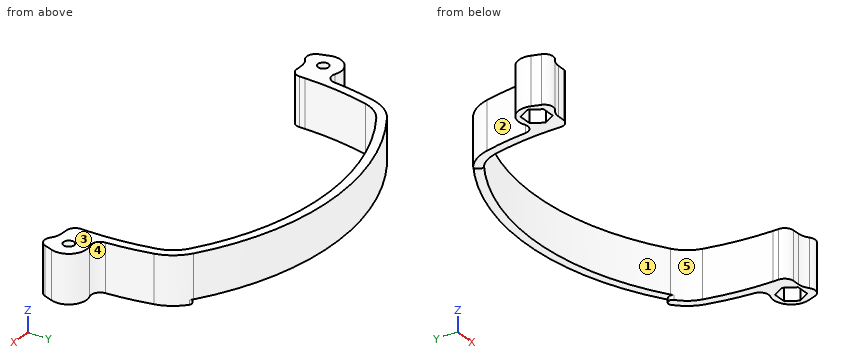
from build123d import *

# Parameters (mm, degrees)
BOSS_EXTRUDE1_DEPTH   = 17.145
BOSS_EXTRUDE2_START   = -17.145
BOSS_EXTRUDE2_DEPTH   = 17.145
F_6_CLEARANCE_HOLE3_D = 3.7973
CUT_EXTRUDE2_DEPTH    = 6.35
FILLET1_R             = 3.175
CUT_EXTRUDE3_DEPTH    = 1.5875
FILLET2_R             = 1.27


with BuildPart() as part:
    # Sketch1 → Boss-Extrude1 (new body)
    with BuildSketch(Plane.XY):
        with BuildLine():
            Line((-60.325, -44.9072), (-57.15, -44.9072))
            ThreePointArc((-57.15, -44.9072), (-56.454091105, -33.036041743), (-54.37589767, -21.327506412))
            ThreePointArc((-54.37589767, -21.327506412), (-52.38952724, -16.938887877), (-48.911621193, -13.605749768))
            ThreePointArc((-48.911621193, -13.605749768), (0, 0.8128), (48.911621193, -13.605749768))
            ThreePointArc((48.911621193, -13.605749768), (52.38952724, -16.938887877), (54.37589767, -21.327506412))
            ThreePointArc((54.37589767, -21.327506412), (56.454091105, -33.036041743), (57.15, -44.9072))
            Line((57.15, -44.9072), (60.325, -44.9072))
            ThreePointArc((60.325, -44.9072), (59.607343952, -32.665068047), (57.464206972, -20.590640987))
            ThreePointArc((57.464206972, -20.590640987), (54.981243935, -15.104867818), (50.633861375, -10.938445182))
            ThreePointArc((50.633861375, -10.938445182), (0, 3.9878), (-50.633861375, -10.938445182))
            ThreePointArc((-50.633861375, -10.938445182), (-54.981243935, -15.104867818), (-57.464206972, -20.590640987))
            ThreePointArc((-57.464206972, -20.590640987), (-59.607343952, -32.665068047), (-60.325, -44.9072))
        make_face()
    extrude(amount=BOSS_EXTRUDE1_DEPTH)

    # Sketch5 → Boss-Extrude2 (add)
    with BuildSketch(Plane.XY.offset(17.145).offset(BOSS_EXTRUDE2_START)):
        with BuildLine():
            Line((-72.692160527, -46.93606155), (-71.648700283, -50.030736885))
            ThreePointArc((-71.648700283, -50.030736885), (-69.548845385, -52.05848349), (-66.680845425, -51.514679193))
            ThreePointArc((-66.680845425, -51.514679193), (-64.835115794, -50.509265825), (-62.762296236, -50.16142536))
            Line((-62.762296236, -50.16142536), (-60.304367197, -50.16142536))
            ThreePointArc((-60.304367197, -50.16142536), (-58.037136322, -49.209101486), (-57.129992434, -46.923418531))
            ThreePointArc((-57.129992434, -46.923418531), (-57.144997985, -45.9153589), (-57.15, -44.9072))
            Line((-57.15, -44.9072), (-60.325, -44.9072))
            ThreePointArc((-60.325, -44.9072), (-67.702990917, -38.640962319), (-72.692160527, -46.93606155))
        make_face()
    boss_extrude2 = extrude(amount=BOSS_EXTRUDE2_DEPTH)

    # #6 Clearance Hole3 (through all)
    with Locations(Plane(origin=(0, 0, 0), x_dir=(-1, 0, 0), z_dir=(0, 0, -1))):
        with Locations((66.675, -44.9072)):
            f_6_clearance_hole3 = Hole(F_6_CLEARANCE_HOLE3_D / 2)

    # Sketch9 → Cut-Extrude2 (cut)
    with BuildSketch(Plane(origin=(0, 0, 0), x_dir=(-1, 0, 0), z_dir=(0, 0, -1))):
        Polygon((69.076344107, -40.74795), (64.273655893, -40.74795), (61.872311786, -44.9072), (64.273655893, -49.06645), (69.076344107, -49.06645), (71.477688214, -44.9072), align=None)
    cut_extrude2 = extrude(amount=-CUT_EXTRUDE2_DEPTH, mode=Mode.SUBTRACT)

    # Mirror1: Boss-Extrude2, #6 Clearance Hole3, Cut-Extrude2 across plane
    add(boss_extrude2.mirror(Plane(origin=(0, 0, 0), x_dir=(0, 0, 1), z_dir=(1, 0, 0))))
    add(f_6_clearance_hole3.mirror(Plane(origin=(0, 0, 0), x_dir=(0, 0, 1), z_dir=(1, 0, 0))), mode=Mode.SUBTRACT)
    add(cut_extrude2.mirror(Plane(origin=(0, 0, 0), x_dir=(0, 0, 1), z_dir=(1, 0, 0))), mode=Mode.SUBTRACT)

    # Fillet1
    # the kernel refuses this fillet: 3.175 mm, written as the material it adds along each edge
    with BuildSketch(Plane(origin=(60.325, -44.9072, 0), x_dir=(0.5606119105814275, 0.8280786712107985, 0), z_dir=(0, 0, 1))) as fillet1_piece_1:
        with BuildLine():
            CenterArc((8.89971408, 2.629149781), FILLET1_R, 128.797238818, 107.104635177)
            Line((6.910366227, 5.103643693), (6.87057927, 5.153133571))
            ThreePointArc((6.87057927, 5.153133571), (3.469787737, 2.532047093), (-0.035598856, 0.052582996))
            Line((-0.035598856, 0.052582996), (0.035598856, -0.052582996))
            ThreePointArc((0.035598856, -0.052582996), (3.559885632, 1.028200438), (7.084172408, -0.052582996))
            Line((7.084172408, -0.052582996), (7.119771264, 0))
        make_face()
    extrude(amount=17.145)
    fillet1_2_edges = [part.edges().sort_by_distance(p)[0] for p in [
        (-60.325, -44.9072, 8.5725),
    ]]
    fillet(fillet1_2_edges, radius=FILLET1_R)

    # Sketch10 → Cut-Extrude3 (cut)
    with BuildSketch(Plane(origin=(0, 0, 0), x_dir=(-1, 0, 0), z_dir=(0, 0, -1))):
        with BuildLine():
            Line((-50.633861375, -10.938445182), (-48.911621193, -13.605749768))
            ThreePointArc((-48.911621193, -13.605749768), (0, 0.8128), (48.911621193, -13.605749768))
            Line((48.911621193, -13.605749768), (50.633861375, -10.938445182))
            ThreePointArc((50.633861375, -10.938445182), (0, 3.9878), (-50.633861375, -10.938445182))
        make_face()
    extrude(amount=-CUT_EXTRUDE3_DEPTH, mode=Mode.SUBTRACT)

    # Fillet2
    fillet2_edges = [part.edges().sort_by_distance(p)[0] for p in [
        (50.633861375, -10.938445182, 0.79375),
        (-50.633861375, -10.938445182, 0.79375),
        (-48.911621193, -13.605749768, 0.79375),
        (48.911621193, -13.605749768, 0.79375),
    ]]
    fillet(fillet2_edges, radius=FILLET2_R)


solid = part.part
Build history of the part. All positions in model axes, mm. Face numbers are marked on the shaded views. A direction names the side the tool comes from. Coordinates: 2 decimals unless noted, no trailing zeros. Order: outer loops, then holes, each group sorted by start corner. A loop starts at its lowest first (then second) coordinate and runs counter-clockwise, first axis right, second up. Notation, with made-up numbers: (-20.5, 48) - (-12.5, 48) arc R20 cw to (-12.5, 62) - close; hole circle Ø4 at (-34.5, 2). An arc over 180 degrees is marked (long way). Put each result on its own line as item: value.
1. Saw through at D-D (z = 13.75). Give the number of separate pieces and of enclosed holes in the cut face, and give its area (3 significant figures).
Answer sheet:
separate pieces: 1
enclosed holes: 2
area: 852 mm^2
2. Saw through at A-A (y = -30). Write the cut outline in (x, z) (3 decimals).
Answer sheet:
outline: (-59.259, 0) - (-56.05, 0) - (-56.05, 17.145) - (-59.259, 17.145) - close; (56.05, 0) - (59.259, 0) - (59.259, 17.145) - (56.05, 17.145) - close
3. Saw through at B-B (y = -23.5). Write the cut outline in (x, z) (3 decimals).
Answer sheet:
outline: (-58.115, 0) - (-54.869, 0) - (-54.869, 17.145) - (-58.115, 17.145) - close; (54.869, 0) - (58.115, 0) - (58.115, 17.145) - (54.869, 17.145) - close
4. Drop flat-ended pins along their axis: P1, Ø1, axis at x = -19.5, z = 10, coming from the +Y side; P2, Ø2.5, axis at x = -67, z = 4, coming from the -Y side; P3, Ø0.7, axis at x = 61.5, z = 10, coming from the -Y side; P4, Ø10, axis at y = -46.5, z = 12, coming from the +X side (3 decimals). Give the stop position or say it passes through.
Answer sheet:
P1: stops at y = 2.03
P2: stops at y = -52.17
P3: stops at y = -50.16
P4: stops at x = 73.025
5. Pull direction X, two halves, no side cores. Call the marked faces 1, 2 and 3: pulls with the +X half, pulls with the -X half, needs draft (parallel to the pull), parting line crosses it, or undercut.
Answer sheet:
face 1: undercut
face 2: pulls with the -X half
face 3: needs draft
6. Saw through at C-C (x = -4). Write the cut outline in (y, z) (1 decimal), and give its area (3 significant figures).
Answer sheet:
outline: (0.7, 1.6) - (3.9, 1.6) - (3.9, 17.1) - (0.7, 17.1) - close
area: 49.4 mm^2
7. Probe line 1 along X through (y, z) = (-47, 13.5); line 2 along X through (y, z) = (-12, 9); line 3 along Y through (x, z) = (67, 2). List the from-to ranges inside material, lowest first. Write a range as [from, to].
Answer sheet:
line 1: x = [-72.67, -57.13], [57.13, 72.67]
line 2: x = [-52.09, -46.33], [46.33, 52.09]
line 3: y = [-51.73, -49.07], [-40.75, -38.57]
8. Tool access for the marked faces 4 and 5: list every direction of +Z, -Z, +X, -X, +Y, -Y with a clear straight run to the whole face (end or side of a thin tool).
Answer sheet:
face 4: +Z, -Z, +Y
face 5: +Z, -Z, -Y
